from build123d import *

# Parameters (mm, degrees)
EXTRUDE_1_DEPTH          = 20
EXTRUDE_1_DEPTH_BACK     = 5
EXTRUDE_2_DEPTH          = 5.5
SKETCH_1_5_R             = 1.5
CUT_EXTRUDE_1_DEPTH      = 4.5
CUT_EXTRUDE_1_DEPTH_BACK = 2
SKETCH_3_R               = 1
CUT_EXTRUDE_2_DEPTH      = 100
FILLET_3_R               = 20
FILLET_8_R               = 4


with BuildPart() as part:
    # 草图1 → 凸台-拉伸1 (new body, two sides)
    with BuildSketch(Plane(origin=(0, 0, 0), x_dir=(1, 0, 0), z_dir=(0, 1, 0))) as extrude_1_sk:
        with BuildLine():
            Line((0, -51.852813742), (0, -52.252813742))
            Line((0, -52.252813742), (9.5, -52.252813742))
            Line((9.5, -52.252813742), (9.5, -70.252813742))
            Line((9.5, -70.252813742), (11.5, -70.252813742))
            Line((11.5, -70.252813742), (11.5, -49.052813742))
            Line((11.5, -49.052813742), (9.5, -47.413831048))
            Line((9.5, -47.413831048), (9.5, -44.41312259))
            Line((9.5, -44.41312259), (0, -44.41312259))
            Line((0, -44.41312259), (0, -47.352813742))
            ThreePointArc((0, -47.352813742), (1.5, -48.852813742), (0, -50.352813742))
            Line((0, -50.352813742), (0, -51.852813742))
        make_face()
    extrude(amount=EXTRUDE_1_DEPTH)
    extrude(extrude_1_sk.sketch, amount=-EXTRUDE_1_DEPTH_BACK)

    # 草图1<7> → 凸台-拉伸2 (add)
    with BuildSketch(Plane(origin=(0, 0, 0), x_dir=(1, 0, 0), z_dir=(0, 1, 0))):
        with BuildLine():
            Line((0, -50.352813742), (0, -51.852813742))
            ThreePointArc((0, -51.852813742), (2.274628745, -50.808846481), (2.966165528, -48.403523125))
            Line((2.966165528, -48.403523125), (9.5, -47.413831048))
            Line((9.5, -47.413831048), (9.5, -44.41312259))
            Line((9.5, -44.41312259), (0, -44.41312259))
            Line((0, -44.41312259), (0, -47.352813742))
            ThreePointArc((0, -47.352813742), (1.5, -48.852813742), (0, -50.352813742))
        make_face()
    extrude(amount=EXTRUDE_2_DEPTH)

    # 草图1<5> → 切除-拉伸1 (cut, two sides)
    with BuildSketch(Plane(origin=(0, 0, 0), x_dir=(1, 0, 0), z_dir=(0, 1, 0))) as cut_extrude_1_sk:
        with BuildLine():
            Line((0, -50.352813742), (0, -51.852813742))
            ThreePointArc((0, -51.852813742), (2.274628745, -50.808846481), (2.966165528, -48.403523125))
            Line((2.966165528, -48.403523125), (9.5, -47.413831048))
            Line((9.5, -47.413831048), (9.5, -44.41312259))
            Line((9.5, -44.41312259), (0, -44.41312259))
            Line((0, -44.41312259), (0, -47.352813742))
            ThreePointArc((0, -47.352813742), (1.5, -48.852813742), (0, -50.352813742))
        make_face()
        with BuildLine():
            Line((0, -26.352813742), (0, -29.352813742))
            Line((0, -29.352813742), (10, -29.352813742))
            ThreePointArc((10, -29.352813742), (12.121320344, -24.231493399), (7, -26.352813742))
            Line((7, -26.352813742), (0, -26.352813742))
        make_face()
        with Locations((10, -26.352813742)):
            Circle(SKETCH_1_5_R, mode=Mode.SUBTRACT)
    extrude(amount=CUT_EXTRUDE_1_DEPTH, mode=Mode.SUBTRACT)
    extrude(cut_extrude_1_sk.sketch, amount=-CUT_EXTRUDE_1_DEPTH_BACK, mode=Mode.SUBTRACT)

    # 草图3 → 切除-拉伸2 (cut)
    with BuildSketch(Plane(origin=(11.5, 0, 0), x_dir=(0, 0, -1), z_dir=(1, 0, 0))):
        with BuildLine():
            Line((-57.918477605, 5.5), (-42.203980761, 5.5))
            Line((-42.203980761, 5.5), (-40.897963641, 24.166318072))
            Line((-40.897963641, 24.166318072), (-83.266559668, 28.095474909))
            Line((-83.266559668, 28.095474909), (-85.239587029, -9.794237843))
            Line((-85.239587029, -9.794237843), (-43.684715074, -5.18920723))
            Line((-43.684715074, -5.18920723), (-42.964099773, 0.151496704))
            Line((-42.964099773, 0.151496704), (-49.918517235, 0.151496704))
            Line((-49.918517235, 0.151496704), (-63.77029754, -3.087900575))
            ThreePointArc((-63.77029754, -3.087900575), (-66.684209706, -1.521268022), (-65.492240114, 1.56489953))
            Line((-65.492240114, 1.56489953), (-57.918477605, 5.5))
        make_face()
        with Locations((-64.339596777, -0.653556379)):
            Circle(SKETCH_3_R)
    extrude(amount=-CUT_EXTRUDE_2_DEPTH, mode=Mode.SUBTRACT)

    # 圆角3
    fillet_3_edges = [part.edges().sort_by_distance(p)[0] for p in [
        (7.152165831, 0.151496704, 49.918517235),
    ]]
    fillet(fillet_3_edges, radius=FILLET_3_R)

    # 圆角8
    fillet_8_edges = [part.edges().sort_by_distance(p)[0] for p in [
        (2.966165528, 2.317894753, 48.403523125),
        (9.5, 5, 47.413831048),
        (10.5, 5.5, 57.918477605),
    ]]
    fillet(fillet_8_edges, radius=FILLET_8_R)

    # 镜向1: part across plane


with BuildPart() as part_1:
    add(part.part)
    add(part.part.mirror(Plane(origin=(0, -5, 0), x_dir=(0, 0, 1), z_dir=(1, 0, 0))))


solid = part_1.part
Verification items for the finished model (mm, model axes). A direction names the side the tool comes from. Coordinates: 2 decimals unless noted, no trailing zeros. Order: outer loops, then holes, each group sorted by start corner. A loop starts at its lowest first (then second) coordinate and runs counter-clockwise, first axis right, second up. Notation, with made-up numbers: M 40.5,40.5 L 96.5,40.5 A7 ccw 96.5,45.5 Z; hole C 59.5,12 d8. An arc over 180 degrees is marked long. One line per item, written item: value. Start each with the question number.
Item 1: Access from +Z, -Z, +X, -X, +Y, -Y to the whole of each face (thin tool, end or side, straight path). Record for faces 4 (the flat face through (9.5, 5, 45)), 5 (the cylindrical face through (3.895, 2.211, 48.735)), 6 (the flat face through (-10.51, 2.24, 48.24)), 7 (the flat face through (10.51, 2.24, 48.24)).
Item 2: Mould release check, pull along Y, two halves, no side actions. Record for faces 1 (the cylindrical face through (10.51, -0.61, 65.34)), 2 (the cylindrical face through (-3.895, 2.211, 48.735)), 3 (the cylindrical face through (10.49, 5.39, 57.88)): released by +Y, released by -Y, zero draft, split by the parting line, or undercut.
Item 3: Gauge pin test, flat ends, axial feed: pin 1 (4 mm diameter, centred on y = -1.5, z = 48, fed in from +X); pin 2 (4 mm diameter, centred on x = -6, y = 3.5, fed in from +Z); pin 3 (0.5 mm diameter, centred on y = 5, z = 45, fed in from +X); pin 4 (3.5 mm diameter, centred on x = 3.5, z = 48, fed in from -Y). Record the tip position at first contact, or that the pin passes through.
Item 4: Sectioned sample at D-D (y = 2.5). Enter the section's corners in (x, z).
Item 5: Scan lines: probe 1 along Z at (x, y) = (0, 5.1); probe 2 along X at (y, z) = (1, 57); probe 3 along Z at (x, y) = (0, 3.25). Record each from-to range of solid material in increasing order.
Item 6: Sectioned sample at C-C (z = 59.25). Enter the section's corners in (x, y).
Item 7: Sectioned sample at B-B (y = -1). Enter the section's corners in (x, z), then the cut area to 3 significant figures.
Item 8: Sectioned sample at A-A (z = 55). Enter the section's corners in (x, y).
Conclusion:
1. face 4: -Z, +X, +Y, -Y
1. face 5: -Z, -Y
1. face 6: -Z, -X, -Y
1. face 7: -Z, +X, -Y
2. face 1: undercut
2. face 2: zero draft
2. face 3: released by +Y
3. pin 1: stops at x = 11.5
3. pin 2: stops at z = 52.25
3. pin 3: stops at x = 9.5
3. pin 4: stops at y = 0.04
4. outline: M -11.5,49.05 L -9.5,47.41 L -5.68,47.99 A4 ccw -2.69,50.18 A3 cw 2.69,50.18 A4 ccw 5.68,47.99 L 9.5,47.41 L 11.5,49.05 L 11.5,63.69 L 9.5,63.69 L 9.5,52.25 L -9.5,52.25 L -9.5,63.69 L -11.5,63.69 Z
5. probe 1: z = 44.41 to 47.35, 50.35 to 52.25
5. probe 2: x = -11.5 to -9.5, 9.5 to 11.5
5. probe 3: z = 51.85 to 52.25
6. outline: M -11.5,-2.03 L -9.5,-2.03 L -9.5,4.81 L -11.5,4.81 Z; M 9.5,-2.03 L 11.5,-2.03 L 11.5,4.81 L 9.5,4.81 Z
7. outline: M -11.5,54.84 L -9.5,54.84 L -9.5,63.4 L -11.5,63.4 Z; M -11.5,65.28 L -9.5,65.28 L -9.5,66.82 L -11.5,66.82 Z; M 9.5,54.84 L 11.5,54.84 L 11.5,63.4 L 9.5,63.4 Z; M 9.5,65.28 L 11.5,65.28 L 11.5,66.82 L 9.5,66.82 Z
7. area: 40.4 mm^2
8. outline: M -11.5,-1.04 L -9.5,-1.04 L -9.5,5.5 L -11.5,5.5 Z; M 9.5,-1.04 L 11.5,-1.04 L 11.5,5.5 L 9.5,5.5 Z
